from build123d import *

# Parameters (mm, degrees)
F0_R     = 11.2
F1_DEPTH = 7
F2_R     = 1.5


with BuildPart() as f1:
    # F0 (on Top) → F1 (new body)
    with BuildSketch(Plane.XY):
        Polygon((-29.469332, 26.720898), (-12.492945, 30.983096), (-17.749237, 15.576357), (-23.179901, 16.234838), (-20.629681, 11.910552), (-25.649733, 11.956964), (-22.364139, 7.583111), (-33.07862, -4.67234), (-37.875643, 12.160741), (-46.611124, 0.417446), (-46.738951, -13.408707), (-43.685134, -18.698073), (-45.091842, -26.033787), (-38.035573, -28.483399), (-34.981756, -33.772766), (-22.944043, -40.57514), (-8.406311, -38.881639), (-20.585675, -26.310756), (-4.614902, -23.159468), (-2.469832, -28.191802), (0, -23.821104), (2.469832, -28.191802), (4.614902, -23.159468), (20.585675, -26.310756), (8.406311, -38.881639), (22.944043, -40.57514), (34.981756, -33.772766), (38.035573, -28.483399), (45.091842, -26.033787), (43.685134, -18.698073), (46.738951, -13.408707), (46.611124, 0.417446), (37.875643, 12.160741), (33.07862, -4.67234), (22.364139, 7.583111), (25.649733, 11.956964), (20.629681, 11.910552), (23.179901, 16.234838), (17.749237, 15.576357), (12.492945, 30.983096), (29.469332, 26.720898), (23.66708, 40.157694), (11.757195, 47.181472), (5.649561, 47.181472), (0, 52.067574), (-5.649561, 47.181472), (-11.757195, 47.181472), (-23.66708, 40.157694), align=None)
        with Locations((-23.140977, -13.360449)):
            Circle(F0_R, mode=Mode.SUBTRACT)
        with Locations((23.140977, -13.360449)):
            Circle(F0_R, mode=Mode.SUBTRACT)
        Circle(F0_R, mode=Mode.SUBTRACT)
        with Locations((0, 26.720898)):
            Circle(F0_R, mode=Mode.SUBTRACT)
    extrude(amount=F1_DEPTH)

    # F2
    f2_edges = [f1.edges().sort_by_distance(p)[0] for p in [
        (20.981138, 28.851997, 7),
        (26.568206, 33.439296, 7),
        (17.712138, 43.669583, 7),
        (8.703378, 47.181472, 7),
        (2.824781, 49.624523, 7),
        (-8.703378, 47.181472, 7),
        (-17.712138, 43.669583, 7),
        (-26.568206, 33.439296, 7),
        (-20.981138, 28.851997, 7),
        (-15.121091, 23.279726, 7),
        (-20.464569, 15.905597, 7),
        (-27.72138, 1.455386, 7),
        (-23.139707, 11.933758, 7),
        (-21.904791, 14.072695, 7),
        (-24.006936, 9.770038, 7),
        (-35.477131, 3.7442, 7),
        (-42.243383, 6.289093, 7),
        (-46.675037, -6.49563, 7),
        (-45.212043, -16.05339, 7),
        (-44.388488, -22.36593, 7),
        (-41.563707, -27.258593, 7),
        (-28.9629, -37.173953, 7),
        (-15.675177, -39.72839, 7),
        (-36.508664, -31.128083, 7),
        (-14.495993, -32.596197, 7),
        (-12.600289, -24.735112, 7),
        (-3.542367, -25.675635, 7),
        (12.600289, -24.735112, 7),
        (14.495993, -32.596197, 7),
        (3.542367, -25.675635, 7),
        (15.675177, -39.72839, 7),
        (-1.234916, -26.006453, 7),
        (1.234916, -26.006453, 7),
        (28.9629, -37.173953, 7),
        (36.508664, -31.128083, 7),
        (41.563707, -27.258593, 7),
        (44.388488, -22.36593, 7),
        (45.212043, -16.05339, 7),
        (46.675037, -6.49563, 7),
        (42.243383, 6.289093, 7),
        (27.72138, 1.455386, 7),
        (24.006936, 9.770038, 7),
        (20.464569, 15.905597, 7),
        (15.121091, 23.279726, 7),
        (23.139707, 11.933758, 7),
        (21.904791, 14.072695, 7),
        (17.712138, 43.669583, 0),
        (8.703378, 47.181472, 0),
        (2.824781, 49.624523, 0),
        (-8.703378, 47.181472, 0),
        (-17.712138, 43.669583, 0),
        (-2.824781, 49.624523, 0),
        (-26.568206, 33.439296, 0),
        (-15.121091, 23.279726, 0),
        (-20.464569, 15.905597, 0),
        (-35.477131, 3.7442, 0),
    ]]
    fillet(f2_edges, radius=F2_R)


solid = f1.part
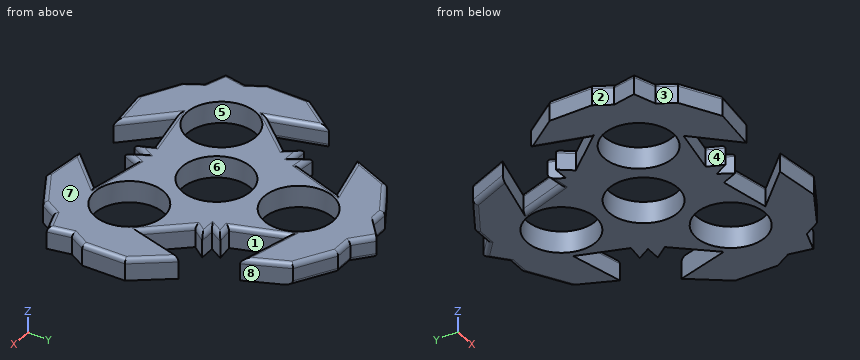
CAD build for the part. Positions are in the model's coordinates, mm. Face numbers are marked on the shaded views. A direction names the side the tool comes from. Round coordinates to 2 decimals unless told otherwise and drop trailing zeros. Use one line per item in the form item = value.
Q1. Flat gauge pins, fed straight in: P1, Ø3, axis at x = 7, y = -23, coming from the +Z side; P2, Ø10, axis at x = -36.5, y = 16, coming from the +Z side; P3, Ø1.2, axis at x = -9.5, z = 4.5, coming from the +Y side; P4, Ø1, axis at y = 2.5, z = 4.5, coming from the +X side. Where does each tip first touch, or does it go through?
Recorded:
P1 = 7
P2 = 6.53
P3 = 47.18
P4 = 45.43
Q2. Saw through at A-A on z = 3.75. State how many separate pieces and enclosed holes the cut face has, then the cut area to 3 significant figures.
Recorded:
separate_pieces = 1
enclosed_holes = 4
area = 3,480 mm^2
Q3. Which spindle directions (+Z, -Z, +X, -X, +Y, -Y) get a long thin tool onto all of the face, cutting with end or side? Do the marked faces 1, 2, 3 and 4. Say none if no direction does.
Recorded:
face_1 = +Z, -Z
face_2 = +Z, -Z, -X
face_3 = +Z, -Z, -X, -Y
face_4 = +Z, -Z, -Y
Q4. Two-plate mould, pull along X, no slides. Class the marked faces 5, 6, 7 and 8: +X half, -X half, draft (parallel to the pull), parting line (faces both ways), or undercut.
Recorded:
face_5 = undercut
face_6 = undercut
face_7 = draft
face_8 = +X half
Q5. Probe L1, parallel to X at y = 0.5, z = 2; L2, parallel to Y at x = 18.5, z = 2.75; L3, parallel to Y at x = 0.5, z = 4.75. List the from-to ranges inside material, lowest first.
Recorded:
L1 = -46.55 to -34.55, -28.56 to -11.19, 11.19 to 28.56, 34.55 to 46.55
L2 = -40.06 to -28.46, -25.9 to -23.55, -3.17 to 15.67, 29.47 to 43.2
L3 = -24.71 to -11.19, 11.19 to 15.53, 37.91 to 51.64
